Work out the finished part from the listing and answer in its coordinate system (mm). A direction names the side the tool comes from. Round coordinates to 2 decimals unless told otherwise and drop trailing zeros. Loops run counter-clockwise (first coordinate to the right, second up) from the corner with the lowest first, then second, coordinate; pieces in that order, holes last.
from build123d import *

# Parameters (mm, degrees)
SKETCH3_W                   = 35
SKETCH3_H                   = 35
SKETCH3_R                   = 5
Y_KSEKLIK_EKSTR_ZYON1_DEPTH = 15
IZIM1_R                     = 5.6
IZIM1_R_2                   = 4.4
KES_EKSTR_ZYON2_DEPTH       = 10
DAIRESEL_KAPLAMA1_COUNT     = 4
KES_EKSTR_ZYON3_DEPTH       = 29.939592257
DAIRESEL_KAPLAMA3_COUNT     = 4
RADYUS3_R                   = 7.5
IZIM4_R                     = 5
IZIM4_R_2                   = 2.5
Y_KSEKLIK_EKSTR_ZYON2_DEPTH = 3


with BuildPart() as part:
    # Sketch3 → Yükseklik-Ekstrüzyon1 (new body)
    with BuildSketch(Plane(origin=(0, 0, 0), x_dir=(1, 0, 0), z_dir=(0, 1, 0))):
        Rectangle(SKETCH3_W, SKETCH3_H)
        with Locations(Location((0, 0, 0), (0, 0, 270))):
            Circle(SKETCH3_R, mode=Mode.SUBTRACT)
    extrude(amount=Y_KSEKLIK_EKSTR_ZYON1_DEPTH)

    # Çizim1 → Kes-Ekstrüzyon2 (cut)
    with BuildSketch(Plane.XY.offset(17.5)):
        with Locations((0, 7.5)):
            Circle(IZIM1_R)
        with Locations((0, 7.5)):
            Circle(IZIM1_R_2, mode=Mode.SUBTRACT)
    kes_ekstr_zyon2 = extrude(amount=-KES_EKSTR_ZYON2_DEPTH, mode=Mode.SUBTRACT)

    # Dairesel Kaplama1: Kes-Ekstrüzyon2 ×4 about axis
    dairesel_kaplama1_axis = Axis((0, 0, 0), (0, 1, 0))
    for i in range(1, DAIRESEL_KAPLAMA1_COUNT):
        add(kes_ekstr_zyon2.rotate(dairesel_kaplama1_axis, i * 360 / DAIRESEL_KAPLAMA1_COUNT), mode=Mode.SUBTRACT)

    # Çizim3 → Kes-Ekstrüzyon3 (cut, through all)
    with BuildSketch(Plane(origin=(0, 15, 0), x_dir=(1, 0, 0), z_dir=(0, 1, 0))):
        with BuildLine():
            ThreePointArc((-6.920403545, -17.5), (-10.019095604, -10.019095604), (-17.5, -6.920403545))
            Line((-17.5, -6.920403545), (-17.5, -17.5))
            Line((-17.5, -17.5), (-6.920403545, -17.5))
        make_face()
    kes_ekstr_zyon3 = extrude(amount=-KES_EKSTR_ZYON3_DEPTH, mode=Mode.SUBTRACT)

    # Dairesel Kaplama3: Kes-Ekstrüzyon3 ×4 about axis
    dairesel_kaplama3_axis = Axis((0, 0, 0), (0, 1, 0))
    for i in range(1, DAIRESEL_KAPLAMA3_COUNT):
        add(kes_ekstr_zyon3.rotate(dairesel_kaplama3_axis, i * 360 / DAIRESEL_KAPLAMA3_COUNT), mode=Mode.SUBTRACT)

    # Radyus3
    # the kernel refuses this fillet: 7.5 mm, written as the material it takes off along each edge
    with BuildSketch(Plane(origin=(-17.5, 15, 17.5), x_dir=(1, 0, 0), z_dir=(0, 0, 1))) as radyus3_piece_1:
        with BuildLine():
            CenterArc((10.579596455 + RADYUS3_R, -RADYUS3_R), RADYUS3_R, 90, 90)
            Line((10.579596455, -RADYUS3_R), (10.579596455 - RADYUS3_R * 0.02, -RADYUS3_R))
            Line((10.579596455 - RADYUS3_R * 0.02, -RADYUS3_R), (10.579596455 - RADYUS3_R * 0.02, RADYUS3_R * 0.02))
            Line((10.579596455 - RADYUS3_R * 0.02, RADYUS3_R * 0.02), (10.579596455 + RADYUS3_R, RADYUS3_R * 0.02))
            Line((10.579596455 + RADYUS3_R, RADYUS3_R * 0.02), (10.579596455 + RADYUS3_R, 0))
        make_face()
    radyus3_piece_1_solid = revolve(axis=Axis((-17.5, 15, 17.5), (0, 1, 0)), revolution_arc=90, mode=Mode.PRIVATE)
    with BuildSketch(Plane(origin=(-17.5, 0, 17.5), x_dir=(1, 0, 0), z_dir=(0, 0, 1))) as radyus3_piece_2:
        with BuildLine():
            CenterArc((10.579596455 + RADYUS3_R, RADYUS3_R), RADYUS3_R, 180, 90)
            Line((10.579596455, RADYUS3_R), (10.579596455 - RADYUS3_R * 0.02, RADYUS3_R))
            Line((10.579596455 - RADYUS3_R * 0.02, RADYUS3_R), (10.579596455 - RADYUS3_R * 0.02, -RADYUS3_R * 0.02))
            Line((10.579596455 - RADYUS3_R * 0.02, -RADYUS3_R * 0.02), (10.579596455 + RADYUS3_R, -RADYUS3_R * 0.02))
            Line((10.579596455 + RADYUS3_R, -RADYUS3_R * 0.02), (10.579596455 + RADYUS3_R, 0))
        make_face()
    radyus3_piece_2_solid = revolve(axis=Axis((-17.5, 0, 17.5), (0, 1, 0)), revolution_arc=90, mode=Mode.PRIVATE)
    with BuildSketch(Plane(origin=(-17.5, 15, -17.5), x_dir=(0, 0, 1), z_dir=(-1, 0, 0))) as radyus3_piece_3:
        with BuildLine():
            CenterArc((10.579596455 + RADYUS3_R, -RADYUS3_R), RADYUS3_R, 90, 90)
            Line((10.579596455, -RADYUS3_R), (10.579596455 - RADYUS3_R * 0.02, -RADYUS3_R))
            Line((10.579596455 - RADYUS3_R * 0.02, -RADYUS3_R), (10.579596455 - RADYUS3_R * 0.02, RADYUS3_R * 0.02))
            Line((10.579596455 - RADYUS3_R * 0.02, RADYUS3_R * 0.02), (10.579596455 + RADYUS3_R, RADYUS3_R * 0.02))
            Line((10.579596455 + RADYUS3_R, RADYUS3_R * 0.02), (10.579596455 + RADYUS3_R, 0))
        make_face()
    radyus3_piece_3_solid = revolve(axis=Axis((-17.5, 15, -17.5), (0, 1, 0)), revolution_arc=90, mode=Mode.PRIVATE)
    with BuildSketch(Plane(origin=(17.5, 15, -17.5), x_dir=(-1, 0, 0), z_dir=(0, 0, -1))) as radyus3_piece_4:
        with BuildLine():
            CenterArc((10.579596455 + RADYUS3_R, -RADYUS3_R), RADYUS3_R, 90, 90)
            Line((10.579596455 + RADYUS3_R, 0), (10.579596455 + RADYUS3_R, RADYUS3_R * 0.02))
            Line((10.579596455 + RADYUS3_R, RADYUS3_R * 0.02), (10.579596455 - RADYUS3_R * 0.02, RADYUS3_R * 0.02))
            Line((10.579596455 - RADYUS3_R * 0.02, RADYUS3_R * 0.02), (10.579596455 - RADYUS3_R * 0.02, -RADYUS3_R))
            Line((10.579596455 - RADYUS3_R * 0.02, -RADYUS3_R), (10.579596455, -RADYUS3_R))
        make_face()
    radyus3_piece_4_solid = revolve(axis=Axis((17.5, 15, -17.5), (0, 1, 0)), revolution_arc=90, mode=Mode.PRIVATE)
    with BuildSketch(Plane(origin=(17.5, 15, 17.5), x_dir=(0, 0, -1), z_dir=(1, 0, 0))) as radyus3_piece_5:
        with BuildLine():
            CenterArc((10.579596455 + RADYUS3_R, -RADYUS3_R), RADYUS3_R, 90, 90)
            Line((10.579596455, -RADYUS3_R), (10.579596455 - RADYUS3_R * 0.02, -RADYUS3_R))
            Line((10.579596455 - RADYUS3_R * 0.02, -RADYUS3_R), (10.579596455 - RADYUS3_R * 0.02, RADYUS3_R * 0.02))
            Line((10.579596455 - RADYUS3_R * 0.02, RADYUS3_R * 0.02), (10.579596455 + RADYUS3_R, RADYUS3_R * 0.02))
            Line((10.579596455 + RADYUS3_R, RADYUS3_R * 0.02), (10.579596455 + RADYUS3_R, 0))
        make_face()
    radyus3_piece_5_solid = revolve(axis=Axis((17.5, 15, 17.5), (0, 1, 0)), revolution_arc=90, mode=Mode.PRIVATE)
    with BuildSketch(Plane(origin=(17.5, 0, 17.5), x_dir=(0, 0, -1), z_dir=(1, 0, 0))) as radyus3_piece_6:
        with BuildLine():
            CenterArc((10.579596455 + RADYUS3_R, RADYUS3_R), RADYUS3_R, 180, 90)
            Line((10.579596455, RADYUS3_R), (10.579596455 - RADYUS3_R * 0.02, RADYUS3_R))
            Line((10.579596455 - RADYUS3_R * 0.02, RADYUS3_R), (10.579596455 - RADYUS3_R * 0.02, -RADYUS3_R * 0.02))
            Line((10.579596455 - RADYUS3_R * 0.02, -RADYUS3_R * 0.02), (10.579596455 + RADYUS3_R, -RADYUS3_R * 0.02))
            Line((10.579596455 + RADYUS3_R, -RADYUS3_R * 0.02), (10.579596455 + RADYUS3_R, 0))
        make_face()
    radyus3_piece_6_solid = revolve(axis=Axis((17.5, 0, 17.5), (0, 1, 0)), revolution_arc=90, mode=Mode.PRIVATE)
    with BuildSketch(Plane(origin=(17.5, 0, -17.5), x_dir=(-1, 0, 0), z_dir=(0, 0, -1))) as radyus3_piece_7:
        with BuildLine():
            CenterArc((10.579596455 + RADYUS3_R, RADYUS3_R), RADYUS3_R, 180, 90)
            Line((10.579596455, RADYUS3_R), (10.579596455 - RADYUS3_R * 0.02, RADYUS3_R))
            Line((10.579596455 - RADYUS3_R * 0.02, RADYUS3_R), (10.579596455 - RADYUS3_R * 0.02, -RADYUS3_R * 0.02))
            Line((10.579596455 - RADYUS3_R * 0.02, -RADYUS3_R * 0.02), (10.579596455 + RADYUS3_R, -RADYUS3_R * 0.02))
            Line((10.579596455 + RADYUS3_R, -RADYUS3_R * 0.02), (10.579596455 + RADYUS3_R, 0))
        make_face()
    radyus3_piece_7_solid = revolve(axis=Axis((17.5, 0, -17.5), (0, 1, 0)), revolution_arc=90, mode=Mode.PRIVATE)
    with BuildSketch(Plane(origin=(-17.5, 0, -17.5), x_dir=(0, 0, 1), z_dir=(-1, 0, 0))) as radyus3_piece_8:
        with BuildLine():
            CenterArc((10.579596455 + RADYUS3_R, RADYUS3_R), RADYUS3_R, 180, 90)
            Line((10.579596455, RADYUS3_R), (10.579596455 - RADYUS3_R * 0.02, RADYUS3_R))
            Line((10.579596455 - RADYUS3_R * 0.02, RADYUS3_R), (10.579596455 - RADYUS3_R * 0.02, -RADYUS3_R * 0.02))
            Line((10.579596455 - RADYUS3_R * 0.02, -RADYUS3_R * 0.02), (10.579596455 + RADYUS3_R, -RADYUS3_R * 0.02))
            Line((10.579596455 + RADYUS3_R, -RADYUS3_R * 0.02), (10.579596455 + RADYUS3_R, 0))
        make_face()
    radyus3_piece_8_solid = revolve(axis=Axis((-17.5, 0, -17.5), (0, 1, 0)), revolution_arc=90, mode=Mode.PRIVATE)
    add([radyus3_piece_1_solid, radyus3_piece_2_solid, radyus3_piece_3_solid, radyus3_piece_4_solid, radyus3_piece_5_solid, radyus3_piece_6_solid, radyus3_piece_7_solid, radyus3_piece_8_solid], mode=Mode.SUBTRACT)

    # Çizim4 → Yükseklik-Ekstrüzyon2 (add)
    with BuildSketch(Plane(origin=(0, 0, 0), x_dir=(1, 0, 0), z_dir=(0, 1, 0))):
        with Locations(Location((0, 0, 0), (0, 0, 270))):
            Circle(IZIM4_R)
        with Locations(Location((0, 0, 0), (0, 0, 270))):
            Circle(IZIM4_R_2, mode=Mode.SUBTRACT)
    extrude(amount=Y_KSEKLIK_EKSTR_ZYON2_DEPTH)


solid = part.part
Item 1: Section B-B, the plane x = 13.5 is taken. State how many separate pieces and enclosed holes the cut face has, plus the area to 3 significant figures.
Item 2: Each of these flat-tipped pins is pushed along its axis until it touches: P1, Ø4, axis at x = 0, z = 0, coming from the -Y side; P2, Ø3, axis at x = -11, z = -6.5, coming from the -Y side; P3, Ø1.5, axis at x = 12.5, z = -5.5, coming from the -Y side. Where does it stop, or does it pass through?
Item 3: Straight lines are drawn through the part: line 1 (Y direction, x = 0, z = 12); line 2 (X direction, y = 1.35, z = 0); line 3 (Z direction, x = -9, y = 5). For each, find the intervals that lie inside material, in ascending order.
Item 4: Section A-A, the plane y = 2.5 is taken. Give the vertices of the cut face in (x, z), plus the area to 3 significant figures.
Item 5: For faces 4 (the face through (-4, 5, 7.5)), 5 (the face through (0.954, 3.205, -12.57)), 6 (the face through (12.57, 2.033, 1.214)), determine the directions among +Z, -Z, +X, -X, +Y, -Y from which every point of the face is accessible in a straight line to the end or side of a thin tool.
Item 6: Determine the mould class of faces 1 (the face through (-12.57, 3.205, -0.954)), 2 (the face through (-6, 7, -17.5)), 3 (the face through (-17.5, 7, 0)) for opening direction Z: pulls with the +Z half, pulls with the -Z half, needs draft (parallel to the pull), parting line crosses it, or undercut.
Answer below:
1. separate pieces: 2
1. enclosed holes: 1
1. area: 142 mm2
2. P1: passes through
2. P2: stops at y = 1.04
2. P3: stops at y = 1.38
3. line 1: y = 0 to 1.9, 3.1 to 11.9, 13.1 to 15
3. line 2: x = -17.5 to -2.5, 2.5 to 17.5
3. line 3: z = -10.5 to -5.01, -3.62 to 3.62, 5.01 to 10.5
4. outline: (-17.5, -5.01) arc R12.49 cw to (-5.01, -17.5) - (-2.52, -17.5) - (-2.52, -7.5) - (2.52, -7.5) - (2.52, -17.5) - (5.01, -17.5) arc R12.49 cw to (17.5, -5.01) - (17.5, -2.52) - (7.5, -2.52) - (7.5, 2.52) - (17.5, 2.52) - (17.5, 5.01) arc R12.49 cw to (5.01, 17.5) - (2.52, 17.5) - (2.52, 7.5) - (-2.52, 7.5) - (-2.52, 17.5) - (-5.01, 17.5) arc R12.49 cw to (-17.5, 5.01) - (-17.5, 2.52) - (-7.5, 2.52) - (-7.5, -2.52) - (-17.5, -2.52) - close; hole circle Ø5 at (0, 0)
4. area: 514 mm2
5. face 4: +Z
5. face 5: -Z
5. face 6: +X
6. face 1: undercut
6. face 2: pulls with the -Z half
6. face 3: needs draft
